```python
from build123d import *

# Parameters (mm, degrees)
BOSS_EXTRU_1_DEPTH      = 5
ESQUISSE2_W             = 20
ESQUISSE2_H             = 5
BOSS_EXTRU_2_DEPTH      = 5
ENL_V_MAT_EXTRU_1_DEPTH = 133.382022949


with BuildPart() as part:
    # Esquisse1 → Boss.-Extru.1 (new body)
    with BuildSketch(Plane.XY):
        Polygon((0, 0), (-100, 0), (-50, 86.602540378), align=None)
    extrude(amount=BOSS_EXTRU_1_DEPTH)

    # Esquisse2 → Boss.-Extru.2 (add)
    with BuildSketch(Plane(origin=(0, 0, 0), x_dir=(-1, 0, 0), z_dir=(0, 0, -1))):
        with Locations((30, -2.5)):
            Rectangle(ESQUISSE2_W, ESQUISSE2_H)
        with Locations((70, -2.5)):
            Rectangle(ESQUISSE2_W, ESQUISSE2_H)
    extrude(amount=-BOSS_EXTRU_2_DEPTH)

    # Esquisse3 → Enlèv. mat.-Extru.1 (cut, through all)
    with BuildSketch(Plane.XY.offset(5)):
        Polygon((-60, 69.282032303), (-55.669872981, 66.782032303), (-65.669872981, 49.461524227), (-70, 51.961524227), align=None)
        Polygon((-80, 34.641016151), (-75.669872981, 32.141016151), (-85.669872981, 14.820508076), (-90, 17.320508076), align=None)
        Polygon((-10, 17.320508076), (-20, 34.641016151), (-24.330127019, 32.141016151), (-14.330127019, 14.820508076), align=None)
        Polygon((-30, 51.961524227), (-40, 69.282032303), (-44.330127019, 66.782032303), (-34.330127019, 49.461524227), align=None)
    extrude(amount=-ENL_V_MAT_EXTRU_1_DEPTH, mode=Mode.SUBTRACT)


solid = part.part
```
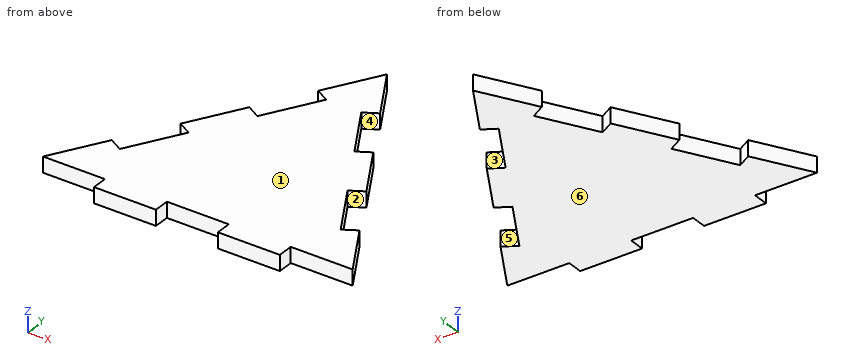
The model under review builds one solid part; all positions refer to its coordinate system, in mm. Face numbers are marked on the shaded views. A direction names the side the tool comes from. Round coordinates to 2 decimals unless told otherwise and drop trailing zeros. Write each loop counter-clockwise with the first axis right and the second up, starting at its lowest first coordinate (ties: lowest second). Pieces come first, ordered by that corner, then holes. Notation, with made-up numbers: (36.25, 56) -> (53.25, 56) arc R23 ccw to (53.25, 83) -> close; hole circle Ø8 at (-32.5, 63.25). An arc over 180 degrees is marked (long way). Use CSV: the item, a comma, the result in double quotes.
Q1. Mouldability with a two-part tool opening along X and no side actions: class the marked faces 1, 2 and 3 as released by +X, released by -X, zero draft, split by the parting line, or undercut.
Checks:
face 1,"zero draft"
face 2,"released by +X"
face 3,"undercut"
Q2. For the marked faces 4, 5 and 6, list the 3-axis set-ups (+Z, -Z, +X, -X, +Y, -Y) from which the entire face can be reached by the end or side of a thin tool; tool diameter is ignored.
Checks:
face 4,"+Z, -Z, +X"
face 5,"+Z, -Z, +Y"
face 6,"-Z, +X, -X, +Y, -Y"
Q3. Consider section C-C (y = 78.5). Give the boundary of the cut face in (x, z), then the cut area to 3 significant figures.
Checks:
outline,"(-54.68, 0) -> (-45.32, 0) -> (-45.32, 5) -> (-54.68, 5) -> close"
area,"46.8 mm²"
Q4. Consider section B-B (x = -26). Give the boundary of the cut face in (y, z).
Checks:
outline,"(-5, 0) -> (45.03, 0) -> (45.03, 5) -> (-5, 5) -> close"
Q5. Consider section A-A (z = 3). Give the boundary of the cut face in (x, y).
Checks:
outline,"(-100, 0) -> (-80, 0) -> (-80, -5) -> (-60, -5) -> (-60, 0) -> (-40, 0) -> (-40, -5) -> (-20, -5) -> (-20, 0) -> (0, 0) -> (-10, 17.32) -> (-14.33, 14.82) -> (-24.33, 32.14) -> (-20, 34.64) -> (-30, 51.96) -> (-34.33, 49.46) -> (-44.33, 66.78) -> (-40, 69.28) -> (-50, 86.6) -> (-60, 69.28) -> (-55.67, 66.78) -> (-65.67, 49.46) -> (-70, 51.96) -> (-80, 34.64) -> (-75.67, 32.14) -> (-85.67, 14.82) -> (-90, 17.32) -> close"
Q6. To check wall thickness, follow probe 1 along X at (y, z) = (16.5, 4.4); probe 2 along Y at (x, z) = (-77, 0.4); probe 3 along Y at (x, z) = (-20.5, 1.9). State the ranges of each line that lie inside material, in increasing order. Write a range as [from, to].
Checks:
probe 1,"[-90.47, -88.58], [-84.7, -15.3], [-11.42, -9.53]"
probe 2,"[-5, 29.84], [32.91, 39.84]"
probe 3,"[-5, 25.51], [34.35, 35.51]"
Q7. For pin 1 Ø1.5 at (x, z) = (-90, 2) entering from -Y; pin 2 Ø1.5 at (y, z) = (-2, 2) entering from -X; pin 3 Ø2 at (x, y) = (-62.5, 70.5) entering from +Z; pin 4 Ø2.5 at (y, z) = (-3.5, 3) entering from +X, all flat-tipped, find the tip position at first contact; note any pin that passes through.
Checks:
pin 1,"y = 0"
pin 2,"x = -80"
pin 3,"through"
pin 4,"x = -20"
